from build123d import *

# Parameters (mm, degrees)
BOSS_EXTRUDE1_DEPTH = 366


with BuildPart() as part:
    # Sketch5 → Boss-Extrude1 (new body)
    with BuildSketch(Plane(origin=(0, 0, 0), x_dir=(0, 0, -1), z_dir=(1, 0, 0))):
        with BuildLine():
            Line((-8.499999996, -2.75), (8.499999996, -2.75))
            Line((8.499999996, -2.75), (8.499999996, 2.25))
            ThreePointArc((8.499999996, 2.25), (8.353553387, 2.603553391), (7.999999996, 2.75))
            Line((7.999999996, 2.75), (5.299999996, 2.75))
            Line((5.299999996, 2.75), (5.299999996, 1.55))
            Line((5.299999996, 1.55), (7.299999998, 1.55))
            Line((7.299999998, 1.55), (7.299999998, 0.05))
            Line((7.299999998, 0.05), (4.249999998, 0.05))
            Line((4.249999998, 0.05), (3.749999998, -0.45))
            Line((3.749999998, -0.45), (0.499999998, -0.45))
            Line((0.499999998, -0.45), (0, -0.738675133))
            Line((0, -0.738675133), (-0.499999998, -0.45))
            Line((-0.499999998, -0.45), (-3.749999998, -0.45))
            Line((-3.749999998, -0.45), (-4.249999998, 0.05))
            Line((-4.249999998, 0.05), (-7.299999998, 0.05))
            Line((-7.299999998, 0.05), (-7.299999998, 1.55))
            Line((-7.299999998, 1.55), (-5.299999996, 1.55))
            Line((-5.299999996, 1.55), (-5.299999996, 2.75))
            Line((-5.299999996, 2.75), (-7.999999996, 2.75))
            ThreePointArc((-7.999999996, 2.75), (-8.353553387, 2.603553391), (-8.499999996, 2.25))
            Line((-8.499999996, 2.25), (-8.499999996, -2.75))
        make_face()
    extrude(amount=BOSS_EXTRUDE1_DEPTH)


solid = part.part
Work out the finished part from the listing and answer in its coordinate system (mm). Round coordinates to 2 decimals unless told otherwise and drop trailing zeros. Write each loop counter-clockwise with the first axis right and the second up, starting at its lowest first coordinate (ties: lowest second). Pieces come first, ordered by that corner, then holes. Notation, with made-up numbers: (37.25, 22.5) -> (45.25, 22.5) arc R23 ccw to (45.25, 53.5) -> close; hole circle Ø1 at (63.25, 30). An arc over 180 degrees is marked (long way). Answer as CSV lines item,"result". Start each with the question number.
(1) Find the intervals of material crossed by probe 1 along Z at (x, y) = (246.5, 0.3); probe 2 along Y at (x, z) = (321, -6); probe 3 along Z at (x, y) = (288, 1.95), in increasing order.
(2) The part is cut by section A-A, the plane x = 240. Give the vertices of the cut face in (y, z).
(3) This flat-tipped pin is pushed along its axis until it touches: pin 1 (1 mm diameter, centred on x = 93, z = -1.5, fed in from +Y). Where does it stop, or does it pass through?
Output values:
1,probe 1,"z = -8.5 to -7.3, 7.3 to 8.5"
1,probe 2,"y = -2.75 to 0.05, 1.55 to 2.75"
1,probe 3,"z = -8.5 to -5.3, 5.3 to 8.5"
2,outline,"(-2.75, -8.5) -> (2.25, -8.5) arc R0.5 ccw to (2.75, -8) -> (2.75, -5.3) -> (1.55, -5.3) -> (1.55, -7.3) -> (0.05, -7.3) -> (0.05, -4.25) -> (-0.45, -3.75) -> (-0.45, -0.5) -> (-0.74, 0) -> (-0.45, 0.5) -> (-0.45, 3.75) -> (0.05, 4.25) -> (0.05, 7.3) -> (1.55, 7.3) -> (1.55, 5.3) -> (2.75, 5.3) -> (2.75, 8) arc R0.5 ccw to (2.25, 8.5) -> (-2.75, 8.5) -> close"
3,pin 1,"stops at y = -0.45"
